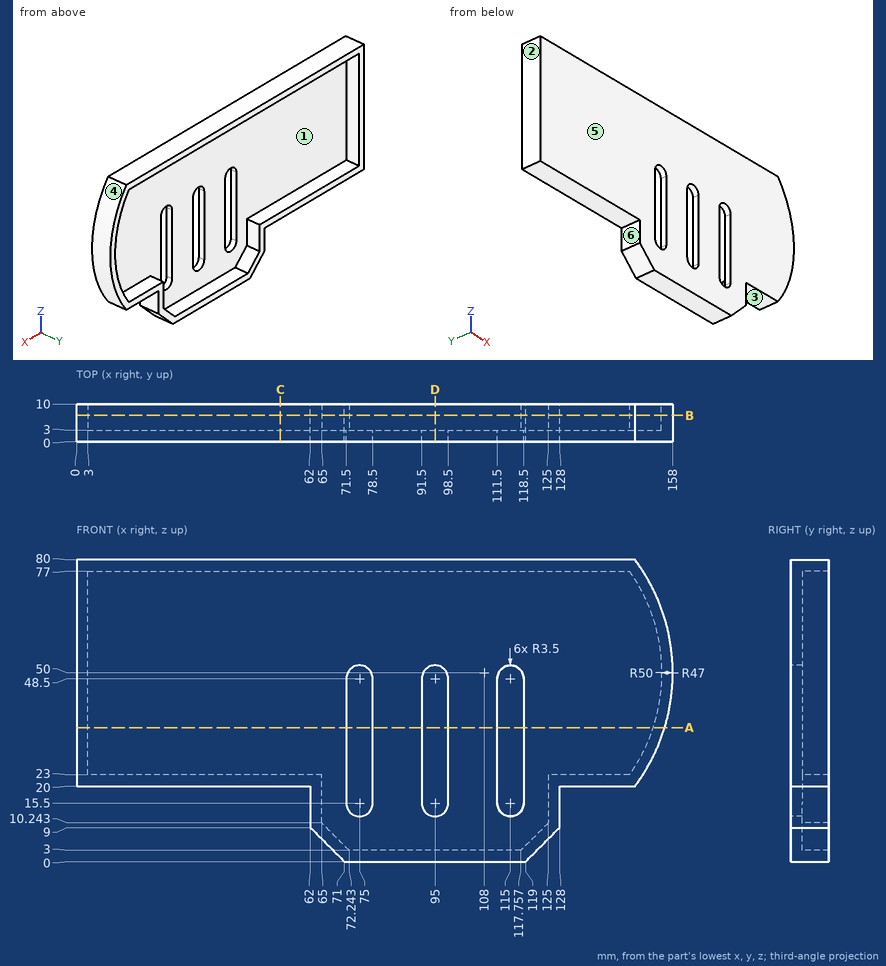
Source: three-view drawing plus pictorial views. Frame: mm from the lowest corner of the part. A direction names the side the tool comes from. Give positions to 0.01 mm unless a question says otherwise; leave off trailing zeros. Loops run counter-clockwise (first coordinate to the right, second up) from the corner with the lowest first, then second, coordinate; pieces in that order, holes last. Notation, with made-up numbers: (42, 18.25) -> (90, 18.25) arc R15 cw to (90, 40.25) -> close; hole circle Ø7 at (12, -14.5). An arc over 180 degrees is marked (long way). Use a Markdown table: item, result. Add a question column.
(1) First-contact query: pin 1 Ø2 at (y, z) = (7.5, 17.5) entering from -X; pin 2 Ø3 at (y, z) = (8.5, 32) entering from +X; pin 3 Ø2 at (y, z) = (6.5, 49) entering from +X. Flat tips, straight axial feed; report the tip coordinate or a pass-through.
(2) Access query for the marked faces 5 and 6. Directions: +Z, -Z, +X, -X, +Y, -Y. A direction counts if a zero-diameter tool reaches every point of the face in a straight line with its end or side. Return the directions, or none.
(3) Section query B-B (y = 7). Output: boundary loops of the cut face in (x, z).
(4) Pull-direction query (X, two-part tool) for the marked faces 1, 2, 3 and 4; classes: +X half, -X half, draft (parallel to the pull), parting line (faces both ways), or undercut.
(5) Ray query, line 1 (Z direction, x = 141.5, y = 4.25); line 2 (Z direction, x = 85, y = 3.5); line 3 (X direction, y = 5.75, z = 49.5). Return the intervals inside material, ascending.
(6) Section query C-C (x = 54). Output: boundary loops of the cut face in (y, z).
(7) Section query D-D (x = 95). Output: boundary loops of the cut face in (y, z).
(8) Section query A-A (z = 35.5). Output: boundary loops of the cut face in (x, y).
Checked values:
| question | item | result |
|---|---|---|
| 1 | pin 1 | x = 62 |
| 1 | pin 2 | x = 155.2 |
| 1 | pin 3 | x = 158 |
| 2 | face 5 | +Z, -Z, +X, -X, -Y |
| 2 | face 6 | -Z, -X, +Y, -Y |
| 3 | outline | (0, 20) -> (62, 20) -> (62, 9) -> (71, 0) -> (119, 0) -> (128, 9) -> (128, 20) -> (148, 20) arc R50 ccw to (148, 80) -> (0, 80) -> close; hole (3, 23) -> (65, 23) -> (65, 10.24) -> (72.24, 3) -> (117.76, 3) -> (125, 10.24) -> (125, 23) -> (146.47, 23) arc R47 ccw to (146.47, 77) -> (3, 77) -> close |
| 4 | face 1 | undercut |
| 4 | face 2 | -X half |
| 4 | face 3 | draft |
| 4 | face 4 | +X half |
| 5 | line 1 | 20 to 23, 77 to 80 |
| 5 | line 2 | 0 to 3, 77 to 80 |
| 5 | line 3 | 0 to 3, 155 to 158 |
| 6 | outline | (0, 20) -> (10, 20) -> (10, 23) -> (3, 23) -> (3, 77) -> (10, 77) -> (10, 80) -> (0, 80) -> close |
| 7 | outline | (0, 0) -> (10, 0) -> (10, 3) -> (3, 3) -> (3, 12) -> (0, 12) -> close; (0, 52) -> (3, 52) -> (3, 77) -> (10, 77) -> (10, 80) -> (0, 80) -> close |
| 8 | outline | (0, 0) -> (71.5, 0) -> (71.5, 3) -> (3, 3) -> (3, 10) -> (0, 10) -> close; (78.5, 0) -> (91.5, 0) -> (91.5, 3) -> (78.5, 3) -> close; (98.5, 0) -> (111.5, 0) -> (111.5, 3) -> (98.5, 3) -> close; (118.5, 0) -> (155.85, 0) -> (155.85, 10) -> (152.71, 10) -> (152.71, 3) -> (118.5, 3) -> close |
